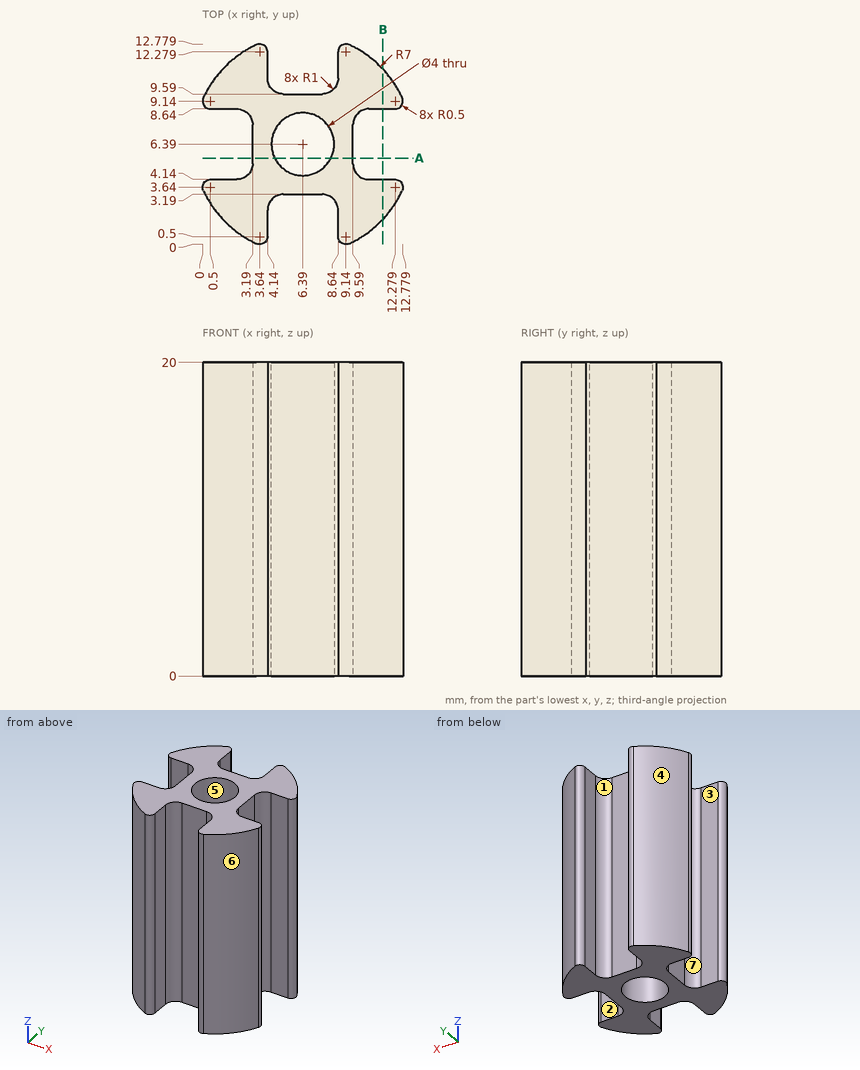
Check sheet for the drawn part. Datum: minimum x, y, z corner. Units: mm. A direction names the side the tool comes from. Round coordinates to 2 decimals unless told otherwise and drop trailing zeros. Order: outer loops, then holes, each group sorted by start corner. A loop starts at its lowest first (then second) coordinate and runs counter-clockwise, first axis right, second up. Notation, with made-up numbers: (1, 6) -> (15, 6) arc R10 cw to (15, 23) -> close; hole circle Ø3 at (48.25, -32.75). An arc over 180 degrees is marked (long way). Put each result on its own line as item: value. Start each with the question number.
(1) Material ranges on line 1 along X through (y, z) = (6.5, 1.75); line 2 along Y through (x, z) = (7.25, 11) (1 decimal); line 3 along X through (y, z) = (11.75, 19.25), recorded low to high.
(2) Draft check along Y on the marked faces 4, 5, 6 and 7. Enter one of: +Y half, -Y half, draft (parallel to the pull), parting line (faces both ways), or undercut.
(3) Depth check by flat-ended pin: pin 1 Ø2 at (y, z) = (8, 5) entering from -X; pin 2 Ø2 at (x, z) = (6, 15) entering from +Y; pin 3 Ø1 at (x, y) = (11, 7.5) entering from -Z; pin 4 Ø0.8 at (x, z) = (1.5, 13.5) entering from -Y. Enter the tip coordinate at first touch or a pass-through.
(4) Section check B-B (x = 11.5). Enter the section's corners in (y, z).
(5) Tool access check on the marked faces 1, 2 and 3. Record the directions out of +Z, -Z, +X, -X, +Y, -Y that give a thin tool (end or side, any length) a straight path to the whole face; none if there is none.
(6) Section check A-A (y = 5.5). Enter the section's corners in (x, z).
Completed:
1. line 1: x = 3.19 to 4.39, 8.39 to 9.59
1. line 2: y = 3.2 to 4.6, 8.2 to 9.6
1. line 3: x = 1.89 to 4.14, 8.64 to 10.89
2. face 4: +Y half
2. face 5: undercut
2. face 6: -Y half
2. face 7: undercut
3. pin 1: stops at x = 0.02
3. pin 2: stops at y = 9.6
3. pin 3: passes through
3. pin 4: stops at y = 1.02
4. outline: (1.61, 0) -> (4.14, 0) -> (4.14, 20) -> (1.61, 20) -> close; (8.64, 0) -> (11.17, 0) -> (11.17, 20) -> (8.64, 20) -> close
5. face 1: +Z, -Z, +Y
5. face 2: +Z, -Z, +X
5. face 3: +Z, -Z, -X
6. outline: (3.19, 0) -> (4.6, 0) -> (4.6, 20) -> (3.19, 20) -> close; (8.18, 0) -> (9.59, 0) -> (9.59, 20) -> (8.18, 20) -> close
